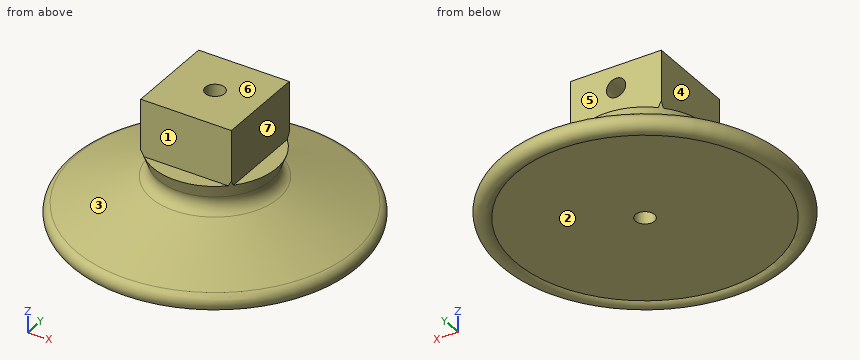
from build123d import *

# Parameters (mm, degrees)
SKETCH3_R                      = 1.5875
CUT_EXTRUDE1_DEPTH             = 1.5000001
CUT_EXTRUDE1_DEPTH_BACK        = 34.456537644
CUT_EXTRUDE2_REACH             = 70.5
SKETCH5_R                      = 1.5875
CUT_EXTRUDE2_DIRECTION_2_DEPTH = 1
CUT_EXTRUDE3_START             = -5.7
SKETCH7_W                      = 73.641561492
SKETCH7_H                      = 95.167537828
SKETCH7_W_2                    = 15
SKETCH7_H_2                    = 15
CUT_EXTRUDE3_DEPTH             = 30
SKETCH8_W                      = 22.620718333
SKETCH8_H                      = 11.010276543
CUT_EXTRUDE4_DEPTH             = 19


with BuildPart() as part:
    # Sketch2 → Revolve1 (revolve)
    with BuildSketch(Plane(origin=(0, 0, 0), x_dir=(0, 0, -1), z_dir=(1, 0, 0))):
        with BuildLine():
            Line((8, 9.378044922), (-13.252418104, 17.371955078))
            ThreePointArc((-13.252418104, 17.371955078), (-15.64910376, 16.565466847), (-15.34, 14.055689912))
            ThreePointArc((-15.34, 14.055689912), (-10.902736423, 7.641374531), (-9.34, 0))
            Line((-9.34, 0), (17.5, 0))
            Line((17.5, 0), (17.5, 21.381966011))
            ThreePointArc((17.5, 21.381966011), (17.339814217, 23.742864466), (15.089610413, 23.010687001))
            Line((15.089610413, 23.010687001), (10.584638888, 10.569083998))
            ThreePointArc((10.584638888, 10.569083998), (9.541151557, 9.433581206), (8, 9.378044922))
        make_face()
    revolve(axis=Axis((0, 0, 9.34), (0, 0, -1)))

    # Sketch6 → Cut-Revolve1 (revolve, cut)
    with BuildSketch(Plane(origin=(0, 0, 0), x_dir=(1, 0, 0), z_dir=(0, 1, 0))):
        Polygon((-15.003814977, -6.956537544), (-14.995054438, -6.959832743), (-17.361955078, -13.252418104), (-17.371955078, -13.252418104), align=None)
    revolve(axis=Axis((0, 0, 0), (0, 0, 1)), mode=Mode.SUBTRACT)

    # Sketch3 → Cut-Extrude1 (cut, two sides)
    with BuildSketch(Plane(origin=(0, 0, -17.5), x_dir=(-1, 0, 0), z_dir=(0, 0, -1))) as cut_extrude1_sk:
        Circle(SKETCH3_R)
    extrude(amount=CUT_EXTRUDE1_DEPTH, mode=Mode.SUBTRACT)
    extrude(cut_extrude1_sk.sketch, amount=-CUT_EXTRUDE1_DEPTH_BACK, mode=Mode.SUBTRACT)

    # Sketch4 → Revolve2 (revolve)
    with BuildSketch(Plane.XY):
        Polygon((0, 1.5875), (5.5, 1.5875), (5.5, 28.5), (4.5, 28.5), (4, 32.5), (4.5, 32.5), (4, 36.5), (4.5, 36.5), (4, 40.5), (4.5, 40.5), (4, 44.5), (0, 44.5), (0, 28.5), align=None)
    revolve(axis=Axis((0, 0, 0), (0, 1, 0)))

    # Sketch5 → Cut-Extrude2 (cut, up to next)
    with BuildSketch(Plane(origin=(0, 44.5, 0), x_dir=(1, 0, 0), z_dir=(0, 1, 0)), mode=Mode.PRIVATE) as cut_extrude2_sk1:
        Circle(SKETCH5_R)
    cut_extrude2_tool1 = extrude(cut_extrude2_sk1.sketch, amount=-CUT_EXTRUDE2_REACH, mode=Mode.PRIVATE) & part.part
    add(cut_extrude2_tool1.solids().sort_by_distance((0, 44.5, 0))[0], mode=Mode.SUBTRACT)

    # Sketch5 → Cut-Extrude2 direction 2 (cut)
    with BuildSketch(Plane(origin=(0, 44.5, 0), x_dir=(1, 0, 0), z_dir=(0, 1, 0))):
        Circle(SKETCH5_R)
    extrude(amount=CUT_EXTRUDE2_DIRECTION_2_DEPTH, mode=Mode.SUBTRACT)

    # Sketch7 → Cut-Extrude3 (cut)
    with BuildSketch(Plane.XY.offset(CUT_EXTRUDE3_START)):
        Rectangle(SKETCH7_W, SKETCH7_H)
        Rectangle(SKETCH7_W_2, SKETCH7_H_2, mode=Mode.SUBTRACT)
    extrude(amount=CUT_EXTRUDE3_DEPTH, mode=Mode.SUBTRACT)

    # Sketch8 → Cut-Extrude4 (cut)
    with BuildSketch(Plane(origin=(0, 7.5, 0), x_dir=(1, 0, 0), z_dir=(0, 1, 0))):
        with Locations((2.733336799, -9.155138272)):
            Rectangle(SKETCH8_W, SKETCH8_H)
    extrude(amount=-CUT_EXTRUDE4_DEPTH, mode=Mode.SUBTRACT)


solid = part.part
Check sheet for the modelled part. Datum: model origin and axes. Units: mm. Face numbers are marked on the shaded views. A direction names the side the tool comes from. Coordinates: 2 decimals unless noted, no trailing zeros. Loops run counter-clockwise (first coordinate to the right, second up) from the corner with the lowest first, then second, coordinate; pieces in that order, holes last. Notation, with made-up numbers: (15, 67) -> (48, 67) arc R9 ccw to (48, 82) -> close; hole circle Ø4 at (73.25, 73). An arc over 180 degrees is marked (long way). Write item = value, one per line. Start each with the question number.
1. Section check B-B on x = 0. Record the cut outline in (y, z), then the cut area to 3 significant figures.
2. Material ranges on line 1 (X direction, y = 2.25, z = 0); line 2 (Z direction, x = 0, y = 3); line 3 (X direction, y = -2, z = 2.5), recorded low to high.
3. Section check A-A on z = 0. Record the cut outline in (x, y) (1 decimal).
4. Tool access check on the marked faces 5, 6 and 7. Record the directions out of +Z, -Z, +X, -X, +Y, -Y that give a thin tool (end or side, any length) a straight path to the whole face; none if there is none.
5. Section check D-D on z = -16.25. Record the cut outline in (x, y) (1 decimal).
6. Draft check along Y on the marked faces 1, 2, 3 and 4. Enter one of: released by +Y, released by -Y, zero draft, split by the parting line, or undercut.
7. Depth check by flat-ended pin: P1, Ø6, axis at y = 8.5, z = -14.5, coming from the +X side; P2, Ø1, axis at x = -3, z = -9, coming from the +Y side; P3, Ø10.5, axis at x = 1, z = -3, coming from the -Y side; P4, Ø5, axis at y = 12.5, z = -2, coming from the -X side (1 decimal). Enter the tip coordinate at first touch or a pass-through.
8. Section check C-C on z = -3. Record the cut outline in (x, y) (1 decimal).
Responses:
q1.outline = (-23.01, -15.09) arc R1.5 ccw (long way) to (-21.38, -17.5) -> (-1.59, -17.5) -> (-1.59, 3.65) -> (-7.5, 3.65) -> (-7.5, -5.7) -> (-10.24, -5.7) -> (-9.38, -8) arc R2 cw to (-10.57, -10.58) -> close; (1.59, -17.5) -> (21.38, -17.5) arc R1.5 ccw (long way) to (23.01, -15.09) -> (10.57, -10.58) arc R2 cw to (9.38, -8) -> (10.24, -5.7) -> (7.5, -5.7) -> (7.5, -1.59) -> (1.59, -1.59) -> close; (1.59, 1.59) -> (7.5, 1.59) -> (7.5, 3.65) -> (1.59, 3.65) -> close
q1.area = 416 mm2
q2.line_1 = -7.5 to -1.59, 1.59 to 7.5
q2.line_2 = -17.5 to -1.59, 1.59 to 3.65
q2.line_3 = -7.5 to 7.5
q3.outline = (-7.5, -7.5) -> (7.5, -7.5) -> (7.5, 7.5) -> (1.6, 7.5) -> (1.6, 0) arc R1.6 cw to (-1.6, 0) -> (-1.6, 7.5) -> (-7.5, 7.5) -> close
q4.face_5 = +Z, +X, -X, +Y
q4.face_6 = +Z, +X, -X, +Y, -Y
q4.face_7 = +Z, +X, +Y, -Y
q5.outline = circle Ø48 at (0, 0); hole circle Ø3.2 at (0, 0)
q6.face_1 = released by -Y
q6.face_2 = undercut
q6.face_3 = split by the parting line
q6.face_4 = zero draft
q7.P1 = 23.2
q7.P2 = 8.98
q7.P3 = -10.24
q7.P4 = through
q8.outline = (-7.5, -7.5) -> (7.5, -7.5) -> (7.5, 7.5) -> (-7.5, 7.5) -> close; hole circle Ø3.2 at (0, 0)
